Geometry check sheet. Reference: drawing and pictorial views, mm from the part's lowest x, y, z. Round coordinates to 2 decimals unless told otherwise and drop trailing zeros. Write each loop counter-clockwise with the first axis right and the second up, starting at its lowest first coordinate (ties: lowest second). Pieces come first, ordered by that corner, then holes. Notation, with made-up numbers: (-33.75, 42.25) -> (1.25, 42.25) arc R26 ccw to (1.25, 56.25) -> close; hole circle Ø8 at (-27, 28). An arc over 180 degrees is marked (long way). Write item = value, one per line.
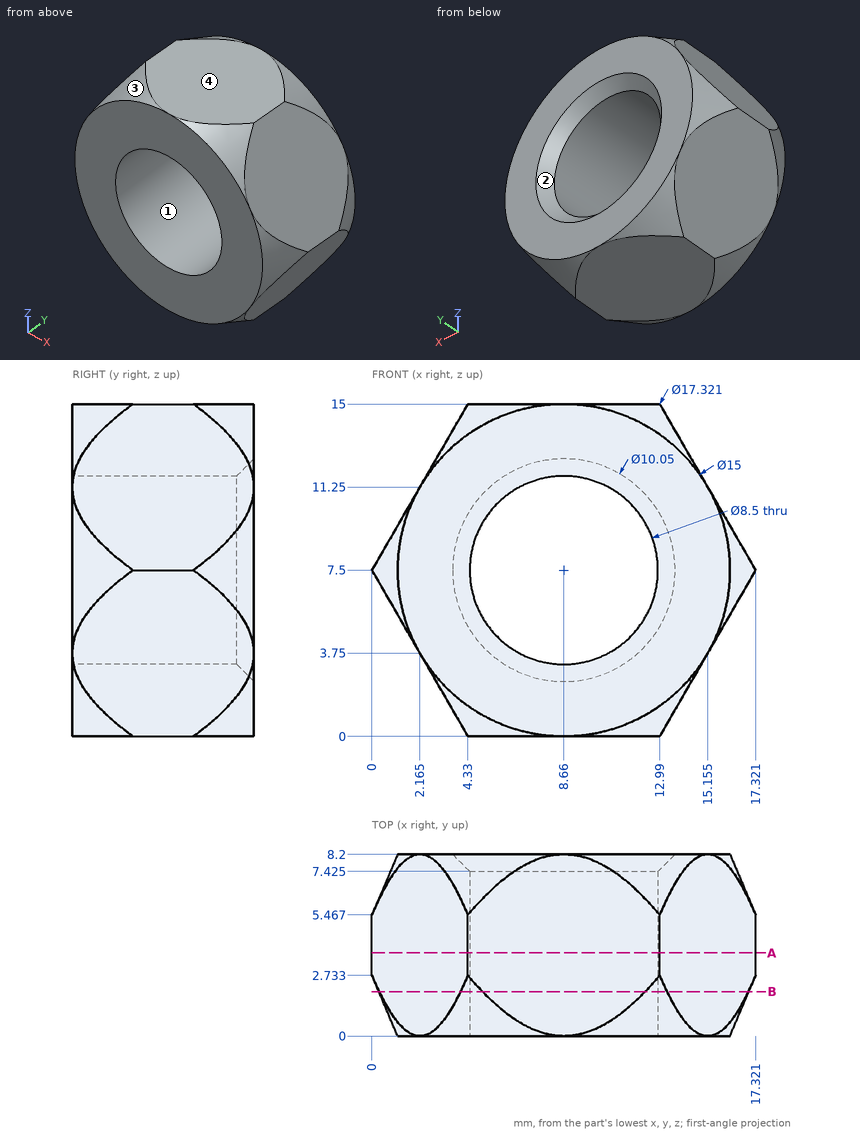
(1) Sectioned sample at B-B on y = 2. Enter the section's corners in (x, z).
Worked answers:
outline = (0.33, 6.93) -> (4, 0.57) arc R8.35 ccw to (4.99, 0) -> (12.33, 0) arc R8.35 ccw to (13.32, 0.57) -> (16.99, 6.93) arc R8.35 ccw to (16.99, 8.07) -> (13.32, 14.43) arc R8.35 ccw to (12.33, 15) -> (4.99, 15) arc R8.35 ccw to (4, 14.43) -> (0.33, 8.07) arc R8.35 ccw to start; hole circle Ø8.5 at (8.66, 7.5)
(2) Material ranges on L1, parallel to Z at x = 12, y = 5 (1 decimal); L2, parallel to Z at x = 12, y = 1 (1 decimal); L3, parallel to Y at x = 4.25, z = 0.5 (1 decimal), recorded low to high. Write a range as [from, to].
Worked answers:
L1 = [0, 4.9], [10.1, 15]
L2 = [0.3, 4.9], [10.1, 14.7]
L3 = [1.8, 6.4]
(3) Go/stop test with flat-tipped pins: P1, Ø2, axis at x = 9.5, z = 6.5, coming from the -Y side; P2, Ø1.5, axis at y = 1.5, z = 3, coming from the +X side (1 decimal). Record where each tip stops, or that it passes through.
Worked answers:
P1 = through
P2 = 15.2
(4) Release check for a two-part mould opening along X. For the marked faces 1, 2, 3 and 4 record: pulls with the +X half, pulls with the -X half, needs draft (parallel to the pull), parting line crosses it, or undercut.
Worked answers:
face_1 = undercut
face_2 = undercut
face_3 = pulls with the -X half
face_4 = needs draft
(5) Sectioned sample at A-A on y = 3.75. Enter the section's corners in (x, z).
Worked answers:
outline = (0, 7.5) -> (4.33, 0) -> (12.99, 0) -> (17.32, 7.5) -> (12.99, 15) -> (4.33, 15) -> close; hole circle Ø8.5 at (8.66, 7.5)
